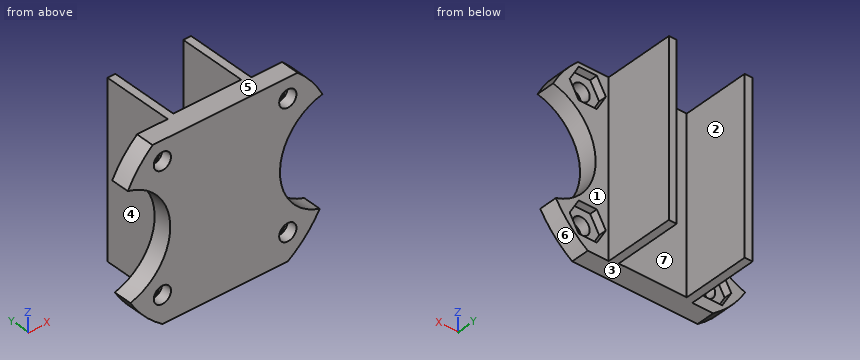
```python
from build123d import *

# Parameters (mm, degrees)
SKETCH1_R               = 21
SKETCH1_R_2             = 1.65
BOSS_EXTRUDE2_DEPTH     = 3.5
CUT_EXTRUDE1_DEPTH      = 1
CUT_EXTRUDE1_DEPTH_BACK = 4.5
BOSS_EXTRUDE3_DEPTH     = 33
CUT_EXTRUDE2_START      = -3.5
CUT_EXTRUDE2_DEPTH      = 1.5
SKETCH7_R               = 10.5
SKETCH7_W               = 41.986856553
SKETCH7_H               = 9.070253879
CUT_EXTRUDE3_DEPTH      = 18


with BuildPart() as part:
    # Sketch1 → Boss-Extrude2 (new body)
    with BuildSketch(Plane(origin=(0, 0, 0), x_dir=(1, 0, 0), z_dir=(0, 1, 0))):
        with Locations((-11.755661444, 8.120165848)):
            Circle(SKETCH1_R)
        with Locations((-23.755661444, 20.120165848)):
            Circle(SKETCH1_R_2, mode=Mode.SUBTRACT)
        with Locations((0.244338556, 20.120165848)):
            Circle(SKETCH1_R_2, mode=Mode.SUBTRACT)
        with Locations((-23.755661444, -3.879834152)):
            Circle(SKETCH1_R_2, mode=Mode.SUBTRACT)
        with Locations((0.244338556, -3.879834152)):
            Circle(SKETCH1_R_2, mode=Mode.SUBTRACT)
    extrude(amount=BOSS_EXTRUDE2_DEPTH)

    # Sketch3 → Cut-Extrude1 (cut, two sides)
    with BuildSketch(Plane(origin=(0, 3.5, 0), x_dir=(1, 0, 0), z_dir=(0, 1, 0))) as cut_extrude1_sk:
        Polygon((-134.766846833, 25.353853788), (-23.755661444, 25.353853788), (0.244338556, 25.353853788), (111.255523946, 25.353853788), (111.255523946, 247.376224567), (-134.766846833, 247.376224567), align=None)
    extrude(amount=CUT_EXTRUDE1_DEPTH, mode=Mode.SUBTRACT)
    extrude(cut_extrude1_sk.sketch, amount=-CUT_EXTRUDE1_DEPTH_BACK, mode=Mode.SUBTRACT)

    # Sketch4 → Boss-Extrude3 (add)
    with BuildSketch(Plane(origin=(0, 0, -25.353853788), x_dir=(-1, 0, 0), z_dir=(0, 0, -1))):
        Polygon((3.755661444, 13.225065807), (3.755661444, 3.5), (19.755661444, 3.5), (19.755661444, 13.225065807), (19.755661444, 17), (18.255661444, 17), (18.255661444, 4), (5.255661444, 4), (5.255661444, 17), (3.755661444, 17), align=None)
    extrude(amount=-BOSS_EXTRUDE3_DEPTH)

    # Sketch6 → Cut-Extrude2 (cut)
    with BuildSketch(Plane.XZ.offset(CUT_EXTRUDE2_START)):
        Polygon((-22.023610636, -17.120165848), (-25.487712251, -17.120165848), (-27.219763059, -20.120165848), (-25.487712251, -23.120165848), (-22.023610636, -23.120165848), (-20.291559828, -20.120165848), align=None)
        Polygon((-22.023610636, 0.879834152), (-20.291559828, 3.879834152), (-22.023610636, 6.879834152), (-25.487712251, 6.879834152), (-27.219763059, 3.879834152), (-25.487712251, 0.879834152), align=None)
        Polygon((1.976389364, 0.879834152), (3.708440172, 3.879834152), (1.976389364, 6.879834152), (-1.487712251, 6.879834152), (-3.219763059, 3.879834152), (-1.487712251, 0.879834152), align=None)
        Polygon((1.976389364, -17.120165848), (-1.487712251, -17.120165848), (-3.219763059, -20.120165848), (-1.487712251, -23.120165848), (1.976389364, -23.120165848), (3.708440172, -20.120165848), align=None)
    extrude(amount=CUT_EXTRUDE2_DEPTH, mode=Mode.SUBTRACT)

    # Sketch7 → Cut-Extrude3 (cut, through all)
    with BuildSketch(Plane.XZ):
        with Locations((-32.749417947, -8.63220869)):
            Circle(SKETCH7_R)
        with Locations((9.237438606, -8.658450465)):
            Circle(SKETCH7_R)
        with Locations((-11.755989671, 12.181273152)):
            Rectangle(SKETCH7_W, SKETCH7_H)
    extrude(amount=-CUT_EXTRUDE3_DEPTH, mode=Mode.SUBTRACT)


solid = part.part
```
Can you work these out from the model? Positions are in its coordinate system, mm. Face numbers are marked on the shaded views. A direction names the side the tool comes from. Coordinates: 2 decimals unless noted, no trailing zeros. Order: outer loops, then holes, each group sorted by start corner. A loop starts at its lowest first (then second) coordinate and runs counter-clockwise, first axis right, second up.
1. Thinking about a two-plate mould opening in X: for the marked faces 5, 6 and 7, which applies, +X half, -X half, draft (parallel to the pull), parting line (faces both ways), or undercut?
2. For the marked faces 1, 2, 3 and 4, which set-ups out of +Z, -Z, +X, -X, +Y, -Y let a thin tool reach every point of the face, with its end or its side?
3. If we section it at C-C (x = -0.5): Please give me the cut outline in (y, z).
4. If we section it at D-D (z = -5): Please give me the cut outline in (x, y).
5. I need wall thicknesses on line 1 (X direction, y = 15.5, z = 3); line 2 (Y direction, x = 4, z = 1); line 3 (Y direction, x = -12, z = 0.5). Which ranges of each line are inside material? Lowest first, please.
6. If we section it at A-A (y = 6.5): Please give me the cut outline in (x, z).
7. I'm going to push flat-ended pins straight in: pin 1 (4 mm diameter, centred on y = 6, z = -13.5, fed in from -X); pin 2 (1.5 mm diameter, centred on x = -9.5, z = -7, fed in from +Y); pin 3 (5 mm diameter, centred on x = 1.5, z = 4, fed in from +Y). Where does each tip first touch, or does it pass through?
8. If we section it at B-B (z = 3): Please give me the cut outline in (x, y), then the cut area to 3 significant figures.
Entries:
1. face 5: draft
1. face 6: +X half
1. face 7: undercut
2. face 1: +Z, -Z, +X, +Y
2. face 2: +Z, -Z, +Y
2. face 3: -Z, +X, -X, +Y, -Y
2. face 4: +Z, -Z, -X, +Y
3. outline: (0, -25.35) - (3.5, -25.35) - (3.5, -23.12) - (2, -23.12) - (2, -21.59) - (0, -21.59) - close; (0, -18.65) - (2, -18.65) - (2, -17.12) - (3.5, -17.12) - (3.5, -12.59) - (0, -12.59) - close; (0, -4.73) - (3.5, -4.73) - (3.5, 0.88) - (2, 0.88) - (2, 2.41) - (0, 2.41) - close; (0, 5.35) - (2, 5.35) - (2, 6.88) - (3.5, 6.88) - (3.5, 7.65) - (0, 7.65) - close
4. outline: (-22.9, 0) - (-0.6, 0) - (-0.6, 3.5) - (-3.76, 3.5) - (-3.76, 17) - (-5.26, 17) - (-5.26, 4) - (-18.26, 4) - (-18.26, 17) - (-19.76, 17) - (-19.76, 3.5) - (-22.9, 3.5) - close
5. line 1: x = -19.76 to -18.26, -5.26 to -3.76
5. line 2: y = 0 to 3.5
5. line 3: y = 0 to 4
6. outline: (-19.76, -25.35) - (-18.26, -25.35) - (-18.26, 7.65) - (-19.76, 7.65) - close; (-5.26, -25.35) - (-3.76, -25.35) - (-3.76, 7.65) - (-5.26, 7.65) - close
7. pin 1: stops at x = -19.76
7. pin 2: stops at y = 4
7. pin 3: stops at y = 3.5
8. outline: (-29.57, 0) - (-25.15, 0) - (-25.15, 2) - (-26.71, 2) - (-26.71, 3.5) - (-29.57, 3.5) - close; (-22.36, 0) - (-1.15, 0) - (-1.15, 2) - (-2.71, 2) - (-2.71, 3.5) - (-3.76, 3.5) - (-3.76, 17) - (-5.26, 17) - (-5.26, 4) - (-18.26, 4) - (-18.26, 17) - (-19.76, 17) - (-19.76, 3.5) - (-20.8, 3.5) - (-20.8, 2) - (-22.36, 2) - close; (1.64, 0) - (6.06, 0) - (6.06, 3.5) - (3.2, 3.5) - (3.2, 2) - (1.64, 2) - close
8. area: 143 mm2
